Geometry: final body of the model. Coordinates: model frame, mm. Give positions to 0.01 mm unless a question says otherwise; leave off trailing zeros. Loops run counter-clockwise (first coordinate to the right, second up) from the corner with the lowest first, then second, coordinate; pieces in that order, holes last. Notation, with made-up numbers: M 64,27 L 114,27 A14 ccw 114,38 Z; hole C -32,-25 d5. An arc over 180 degrees is marked long. One line per question, with ' | ' between items. Start each with the question number.
from build123d import *

# Parameters (mm, degrees)
F1_DEPTH = 19.05
F3_D     = 8.001
F3_DEPTH = 14.224
F3_TIP   = 2.4037429064
F5_D     = 5.0038
F5_DEPTH = 14.224
F5_TIP   = 1.5032931827


with BuildPart() as f1:
    # F0 (on Right) → F1 (new body)
    with BuildSketch(Plane.YZ):
        with BuildLine():
            Line((304.8, -590.55), (304.8, 590.55))
            Line((304.8, 590.55), (285.3894786878, 590.55))
            ThreePointArc((285.3894786878, 590.55), (279.4412012464, 590.2005500018), (273.5747594562, 589.157007696))
            Line((273.5747594562, 589.157007696), (-304.8, 450.85))
            Line((-304.8, 450.85), (-304.8, 428.625))
            Line((-304.8, 428.625), (-304.8, -590.55))
            Line((-304.8, -590.55), (304.8, -590.55))
        make_face()
    extrude(amount=F1_DEPTH)

    # F3
    with Locations(Plane.YZ.offset(19.05)):
        with Locations((-254, 428.625), (-288.925, 393.7), (-9.525, 428.625), (234.95, 428.625), (-254, 206.375), (-9.525, 206.375), (234.95, 206.375), (295.0947393439, 539.75), (295.0947393439, 387.35), (295.0947393439, 133.35), (295.275, -184.15), (295.275, -438.15), (234.95, -530.225), (-231.775, -530.225), (1.6002, -530.225)):
            Hole(F3_D / 2, depth=F3_DEPTH)
            with Locations((0, 0, -(F3_DEPTH + F3_TIP / 2))):  # 118° drill point
                Cone(0, F3_D / 2, F3_TIP, mode=Mode.SUBTRACT)

    # F5
    with Locations(Plane.YZ.offset(19.05)):
        with Locations((-203.2, 117.475), (-203.2, 85.725), (-203.2, 53.975), (-203.2, 22.225), (-203.2, -9.525), (-203.2, -41.275), (-203.2, -73.025), (-203.2, -104.775), (-203.2, -136.525), (-203.2, -168.275), (-203.2, -200.025), (-203.2, -231.775), (-203.2, -263.525), (-203.2, -295.275), (-203.2, -327.025), (-203.2, -358.775), (-203.2, -390.525), (-203.2, -422.275), (203.2, -422.275), (203.2, -390.525), (203.2, -358.775), (203.2, -327.025), (203.2, -295.275), (203.2, -263.525), (203.2, -231.775), (203.2, -200.025), (203.2, -168.275), (203.2, -136.525), (203.2, -104.775), (203.2, -73.025), (203.2, -41.275), (203.2, -9.525), (203.2, 22.225), (203.2, 53.975), (203.2, 85.725), (203.2, 117.475)):
            Hole(F5_D / 2, depth=F5_DEPTH)
            with Locations((0, 0, -(F5_DEPTH + F5_TIP / 2))):  # 118° drill point
                Cone(0, F5_D / 2, F5_TIP, mode=Mode.SUBTRACT)


solid = f1.part
Q1. Section C-C, the plane y = 37. Output: boundary loops of the cut face in (x, z), plus the area to 3 significant figures.
Q2. Contact query for flat-ended pins moving along their axis: pin 1 (4.5 mm diameter, centred on y = -203.2, z = -422.275, fed in from +X); pin 2 (2 mm diameter, centred on x = 11.5, y = -149, fed in from +Z); pin 3 (7 mm diameter, centred on y = -288.925, z = 393.7, fed in from +X). Output: stop coordinate, or through.
Q3. Section B-B, the plane y = 160. Output: boundary loops of the cut face in (x, z), plus the area to 3 significant figures.
Q4. Section A-A, the plane x = 12.5. Count the separate pieces of the cut face and the enclosed holes in it, plus the area to 3 significant figures.
Q5. Material intervals for L1, parallel to Y at x = 13.5, z = 85.5; L2, parallel to Y at x = 17.5, z = -439; L3, parallel to Y at x = 16.25, z = -184.15, sorted ascending.
Model answer:
1) outline: M 0,-590.55 L 19.05,-590.55 L 19.05,532.58 L 0,532.58 Z | area: 21,400 mm^2
2) pin 1: stops at x = 4.67 | pin 2: stops at z = 488.35 | pin 3: stops at x = 4.53
3) outline: M 0,-590.55 L 19.05,-590.55 L 19.05,562 L 0,562 Z | area: 22,000 mm^2
4) separate pieces: 1 | enclosed holes: 51 | area: 678,000 mm^2
5) L1: y = -304.8 to -205.69, -200.71 to 200.71, 205.69 to 304.8 | L2: y = -304.8 to 291.37, 299.18 to 304.8 | L3: y = -304.8 to 291.27, 299.28 to 304.8
